Autodesk Inventor part; units mm, degrees
ref_plane "YZ Plane" through (0, 0, 0) normal (1, 0, 0) x (0, 1, 0)
ref_plane "XZ Plane" through (0, 0, 0) normal (0, 1, 0) x (-1, 0, 0)
ref_plane "XY Plane" through (0, 0, 0) normal (0, 0, 1) x (1, 0, 0)
sketch "Náčrt1" plane through (0, 0, 0) normal (0, 1, 0) x (-1, 0, 0)
  circle A0 centre (0, 0) radius 115
  circle A1 centre (0, 0) radius 92.5
  circle A2 centre (0, 0) radius 35
  circle A3 centre (0, 0) radius 65
  dimension "d0" = 230
  dimension "d1" = 185
  dimension "d2" = 70
  dimension "d3" = 130
extrude "Vysunutí1" add sketch "Náčrt1" along normal blind 95 contours A3
extrude "Vysunutí2" add sketch "Náčrt1" along normal blind 21 contours A1
extrude "Vysunutí3" add sketch "Náčrt1" along normal blind 45 contours A0
sketch "Náčrt2" plane through (0, 21, 0) normal (0, 1, 0) x (1, 0, 0)
  circle A0 centre (0, 0) radius 65 construction
  line L0 (0, -65) -> (0, -92.5) construction
  circle A1 centre (0, 0) radius 92.5 construction
  circle A2 centre (0, -78.75) radius 8.5
  circle A3 centre (68.1995, -39.375) radius 8.5
  circle A4 centre (68.1995, 39.375) radius 8.5
  circle A5 centre (0, 78.75) radius 8.5
  circle A6 centre (-68.1995, 39.375) radius 8.5
  circle A7 centre (-68.1995, -39.375) radius 8.5
  dimension "d10" = 27.5
  dimension "d11" = 17
  dimension "d14" = 360
extrude "Vysunutí4" cut sketch "Náčrt2" against normal through all
sketch "Náčrt3" plane through (0, 0, 0) normal (0, -1, 0) x (1, 0, 0)
  line L0 (-10, 41) -> (10, 41)
  line L1 (10, 41) -> (10, 29)
  line L2 (10, 29) -> (-10, 29)
  line L3 (-10, 29) -> (-10, 41)
  circle A0 centre (0, 0) radius 35
  line L4 (-10, 41) -> (10, 29) construction
  line L5 (10, 41) -> (-10, 29) construction
  point P0 (0, 35)
  point P1 (0, 29)
  dimension "d18" = 20
  dimension "d19" = 12
  dimension "d20" = 29
extrude "Vysunutí5" cut sketch "Náčrt3" against normal through all contours L0 L1 A0 L3 | A0 L1 L2 L3 picked at (1.1251, 30.9456)
properties part number "projektspojkas2v1" material "Sedá litina"
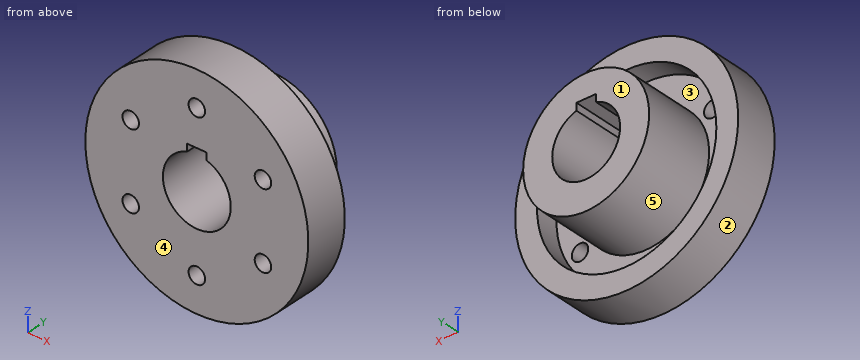
Design review of the part built by this model. Coordinates are the model's own, in mm. Face numbers are marked on the shaded views. A direction names the side the tool comes from. Round coordinates to 2 decimals unless told otherwise and drop trailing zeros. Order: outer loops, then holes, each group sorted by start corner. A loop starts at its lowest first (then second) coordinate and runs counter-clockwise, first axis right, second up. Notation, with made-up numbers: M -28.75,55.5 L -9.75,55.5 A20 cw -9.75,61.5 Z; hole C 38,83 d7. An arc over 180 degrees is marked long. Answer as CSV lines item,"result". Start each with the question number.
1) Add section A-A (x = 0). Give the boundary of the cut face in (y, z), then the cut area to 3 significant figures.
2) Add section C-C (z = 0). Give the boundary of the cut face in (x, y).
3) For pin 1 Ø2 at (y, z) = (47.5, 36) entering from +X; pin 2 Ø8 at (x, y) = (-43, 13) entering from -Z (3 decimals); pin 3 Ø12 at (x, z) = (70, -58.5) entering from +Y, all flat-tipped, find the tip position at first contact; note any pin that passes through.
4) Add section B-B (y = 37). Give the boundary of the cut face in (x, z).
5) Add section D-D (y = 85). Give the boundary of the cut face in (x, z), then the cut area to 3 significant figures.
6) The part is to be moulded in two halves that separate along Z. For the marked faces 1, 2 and 3, say which applies: +Z half, -Z half, draft (parallel to the pull), parting line (faces both ways), or undercut.
7) Wall thickness on line 1 along Z through (x, y) = (0, 35.75); line 2 along Z through (x, y) = (0, 9); line 3 along X through (y, z) = (22, 13): over which ranges is each line inside the solid? List them lowest first. Write a range as [from, to].
8) Tool access review of the marked faces 4 and 5: name each direction out of +Z, -Z, +X, -X, +Y, -Y from which nothing blocks a thin tool from reaching the whole face with its end or side.
Resolved:
1,outline,"M 0,-115 L 45,-115 L 45,-92.5 L 21,-92.5 L 21,-87.25 L 0,-87.25 Z; M 0,-70.25 L 21,-70.25 L 21,-65 L 95,-65 L 95,-35 L 0,-35 Z; M 0,41 L 95,41 L 95,65 L 21,65 L 21,70.25 L 0,70.25 Z; M 0,87.25 L 21,87.25 L 21,92.5 L 45,92.5 L 45,115 L 0,115 Z"
1,area,"7,600 mm^2"
2,outline,"M -115,0 L -35,0 L -35,95 L -65,95 L -65,21 L -92.5,21 L -92.5,45 L -115,45 Z; M 35,0 L 115,0 L 115,45 L 92.5,45 L 92.5,21 L 65,21 L 65,95 L 35,95 Z"
3,pin 1,"x = 54.77"
3,pin 2,"z = -108.185"
3,pin 3,"y = 45"
4,outline,"C 0,0 d230; C 0,0 d130; hole C 0,0 d185; hole M -10,33.54 A35 ccw long 10,33.54 L 10,41 L -10,41 Z"
5,outline,"C 0,0 d130; hole M -10,33.54 A35 ccw long 10,33.54 L 10,41 L -10,41 Z"
5,area,"9,300 mm^2"
6,face 1,"draft"
6,face 2,"parting line"
6,face 3,"undercut"
7,line 1,"[-115, -92.5], [-65, -35], [41, 65], [92.5, 115]"
7,line 2,"[-115, -87.25], [-70.25, -35], [41, 70.25], [87.25, 115]"
7,line 3,"[-114.26, -91.58], [-63.69, -32.5], [32.5, 63.69], [91.58, 114.26]"
8,face 4,"+Z, -Z, +X, -X, -Y"
8,face 5,"+Y"
